from build123d import *

# Parameters (mm, degrees)
EXTRUDE_1_DEPTH     = 10
SKETCH_3_W          = 8
SKETCH_3_H          = 60
EXTRUDE_2_DEPTH     = 72
SKETCH_4_W          = 6
SKETCH_4_H          = 40
EXTRUDE_3_DEPTH     = 16
SKETCH_5_R          = 30
CUT_EXTRUDE_1_DEPTH = 159.962259672
SKETCH_6_R          = 2
CUT_EXTRUDE_2_DEPTH = 10
SKETCH_7_R          = 1.5
CUT_EXTRUDE_3_DEPTH = 10


with BuildPart() as part:
    # 草图1 → 凸台-拉伸1 (new body)
    with BuildSketch(Plane(origin=(0, 0, 0), x_dir=(1, 0, 0), z_dir=(0, 1, 0))):
        with BuildLine():
            Line((-38, -75), (-38, 75))
            ThreePointArc((-38, 75), (0, 113), (38, 75))
            Line((38, 75), (38, -75))
            ThreePointArc((38, -75), (0, -113), (-38, -75))
        make_face()
    extrude(amount=EXTRUDE_1_DEPTH)

    # 草图3 → 凸台-拉伸2 (add)
    with BuildSketch(Plane(origin=(0, 10, 0), x_dir=(1, 0, 0), z_dir=(0, 1, 0))):
        with Locations((-34, -34)):
            Rectangle(SKETCH_3_W, SKETCH_3_H)
        with Locations((34, -34)):
            Rectangle(SKETCH_3_W, SKETCH_3_H)
    extrude(amount=EXTRUDE_2_DEPTH)

    # 草图4 → 凸台-拉伸3 (add)
    with BuildSketch(Plane(origin=(0, 10, 0), x_dir=(1, 0, 0), z_dir=(0, 1, 0))):
        with Locations((-35, 36)):
            Rectangle(SKETCH_4_W, SKETCH_4_H)
        with Locations((35, 36)):
            Rectangle(SKETCH_4_W, SKETCH_4_H)
    extrude(amount=EXTRUDE_3_DEPTH)

    # 草图5 → 切除-拉伸1 (cut, through all)
    with BuildSketch(Plane(origin=(38, 0, 0), x_dir=(0, 0, -1), z_dir=(1, 0, 0))):
        with Locations((-34, 97)):
            Circle(SKETCH_5_R)
    extrude(amount=-CUT_EXTRUDE_1_DEPTH, mode=Mode.SUBTRACT)

    # 草图6 → 切除-拉伸2 (cut)
    with BuildSketch(Plane.XY.offset(64)):
        with Locations((-34, 46)):
            Circle(SKETCH_6_R)
        with Locations((-34, 30)):
            Circle(SKETCH_6_R)
        with Locations((34, 46)):
            Circle(SKETCH_6_R)
        with Locations((34, 30)):
            Circle(SKETCH_6_R)
    extrude(amount=-CUT_EXTRUDE_2_DEPTH, mode=Mode.SUBTRACT)

    # 草图7 → 切除-拉伸3 (cut)
    with BuildSketch(Plane(origin=(0, 26, 0), x_dir=(1, 0, 0), z_dir=(0, 1, 0))):
        with Locations(Location((-35, 26, 0), (0, 0, 270))):
            Circle(SKETCH_7_R)
        with Locations(Location((-35, 46, 0), (0, 0, 270))):
            Circle(SKETCH_7_R)
        with Locations(Location((35, 26, 0), (0, 0, 270))):
            Circle(SKETCH_7_R)
        with Locations(Location((35, 46, 0), (0, 0, 270))):
            Circle(SKETCH_7_R)
    extrude(amount=-CUT_EXTRUDE_3_DEPTH, mode=Mode.SUBTRACT)


solid = part.part
For this review, take the finished solid that the model builds, in its own axes (mm). A direction names the side the tool comes from. Coordinates: 2 decimals unless noted, no trailing zeros. Loops run counter-clockwise (first coordinate to the right, second up) from the corner with the lowest first, then second, coordinate; pieces in that order, holes last. Notation, with made-up numbers: (-7, 72) - (50, 72) arc R21 cw to (50, 78) - close; hole circle Ø6 at (65.25, -18). An arc over 180 degrees is marked (long way). Use a Markdown table: item, result. Add a question column.
Item 1: We need section D-D (x = -6). Give the boundary of the cut face in (y, z), and give its area (3 significant figures).
Item 2: Tool access review of faces 4 (the face through (34.923, 44.226, 59.07)), 5 (the face through (35, 18, -16)), 6 (the face through (-35, 18, -56)), 7 (the face through (37, 45, 64)), 8 (the face through (-30, 37, 34)): name each direction out of +Z, -Z, +X, -X, +Y, -Y from which nothing blocks a thin tool from reaching the whole face with its end or side.
Item 3: For line 1 (Y direction, x = 34, z = 60.75); line 2 (X direction, y = 18.25, z = -46); line 3 (X direction, y = 15.5, z = -22), list the stretches that pass through material, from the lowest coordinate up.
Item 4: We need section C-C (y = 74). Give the boundary of the cut face in (x, z).
Item 5: Insertion check: pin 1 Ø6 at (x, z) = (-21.5, 81.5) entering from +Y; pin 2 Ø2.5 at (x, z) = (-35.5, -25.5) entering from +Y; pin 3 Ø2.5 at (x, z) = (35, -26) entering from +Y. Each pin has a flat end and moves straight along its axis. Give the tip position at first contact, or say it passes through.
Item 6: We need section B-B (z = 38). Give the boundary of the cut face in (x, y).
Item 7: Mouldability with a two-part tool opening along Y and no side actions: class faces 1 (the face through (-33.077, 44.226, 59.07)), 2 (the face through (-34, 67, 34)), 3 (the face through (30, 37, 34)) as pulls with the +Y half, pulls with the -Y half, needs draft (parallel to the pull), parting line crosses it, or undercut.
Item 8: We need section A-A (y = 37.5). Give the boundary of the cut face in (x, z), and give its area (3 significant figures).
Results list:
| question | item | result |
|---|---|---|
| 1 | outline | (0, -112.52) - (10, -112.52) - (10, 112.52) - (0, 112.52) - close |
| 1 | area | 2,250 mm^2 |
| 2 | face 4 | +Z |
| 2 | face 5 | +X, -X, +Y |
| 2 | face 6 | -Z, +X, -X, +Y |
| 2 | face 7 | +Z, +X, -X, +Y |
| 2 | face 8 | +Z, -Z, +Y |
| 3 | line 1 | y = 0 to 28, 32 to 44, 48 to 82 |
| 3 | line 2 | x = -38 to -36.5, -33.5 to -32, 32 to 33.5, 36.5 to 38 |
| 3 | line 3 | x = -38 to -32, 32 to 38 |
| 4 | outline | (-38, 4) - (-30, 4) - (-30, 14.74) - (-38, 14.74) - close; (-38, 53.26) - (-30, 53.26) - (-30, 64) - (-38, 64) - close; (30, 4) - (38, 4) - (38, 14.74) - (30, 14.74) - close; (30, 53.26) - (38, 53.26) - (38, 64) - (30, 64) - close |
| 5 | pin 1 | stops at y = 10 |
| 5 | pin 2 | stops at y = 26 |
| 5 | pin 3 | stops at y = 16 |
| 6 | outline | (-38, 0) - (38, 0) - (38, 67.27) - (30, 67.27) - (30, 10) - (-30, 10) - (-30, 67.27) - (-38, 67.27) - close |
| 7 | face 1 | undercut |
| 7 | face 2 | pulls with the +Y half |
| 7 | face 3 | needs draft |
| 8 | outline | (-38, 4) - (-30, 4) - (-30, 64) - (-38, 64) - close; (30, 4) - (38, 4) - (38, 64) - (30, 64) - close |
| 8 | area | 960 mm^2 |
